```python
from build123d import *

# Parameters (mm, degrees)
F1_DEPTH = 914.4
F2_R     = 19.05
F3_DEPTH = 127
F4_W     = 41.148
F4_H     = 203.2
F5_DEPTH = 127


with BuildPart() as f1:
    # F0 (on Front) → F1 (new body, symmetric)
    with BuildSketch(Plane.XZ):
        with BuildLine():
            ThreePointArc((50.8, 44.45), (48.940128, 48.940128), (44.45, 50.8))
            Line((44.45, 50.8), (-44.45, 50.8))
            ThreePointArc((-44.45, 50.8), (-48.940128, 48.940128), (-50.8, 44.45))
            Line((-50.8, 44.45), (-50.8, -44.45))
            ThreePointArc((-50.8, -44.45), (-48.940128, -48.940128), (-44.45, -50.8))
            Line((-44.45, -50.8), (44.45, -50.8))
            ThreePointArc((44.45, -50.8), (48.940128, -48.940128), (50.8, -44.45))
            Line((50.8, -44.45), (50.8, 44.45))
        make_face()
        with BuildLine():
            Line((-34.925, 41.275), (34.925, 41.275))
            ThreePointArc((34.925, 41.275), (39.415128, 39.415128), (41.275, 34.925))
            Line((41.275, 34.925), (41.275, -34.925))
            ThreePointArc((41.275, -34.925), (39.415128, -39.415128), (34.925, -41.275))
            Line((34.925, -41.275), (-34.925, -41.275))
            ThreePointArc((-34.925, -41.275), (-39.415128, -39.415128), (-41.275, -34.925))
            Line((-41.275, -34.925), (-41.275, 34.925))
            ThreePointArc((-41.275, 34.925), (-39.415128, 39.415128), (-34.925, 41.275))
        make_face(mode=Mode.SUBTRACT)
    extrude(amount=F1_DEPTH, both=True)

    # F2 (on face) → F3 (cut)
    with BuildSketch(Plane.YZ.offset(50.8)):
        with Locations((304.8, 0)):
            Circle(F2_R)
        with Locations((-762, 0)):
            Circle(F2_R)
        with Locations((-609.6, 0)):
            Circle(F2_R)
        with Locations((-457.2, 0)):
            Circle(F2_R)
        with Locations((-304.8, 0)):
            Circle(F2_R)
        with Locations((-152.4, 0)):
            Circle(F2_R)
        Circle(F2_R)
        with Locations((152.4, 0)):
            Circle(F2_R)
        with Locations((457.2, 0)):
            Circle(F2_R)
        with Locations((609.6, 0)):
            Circle(F2_R)
    extrude(amount=-F3_DEPTH, mode=Mode.SUBTRACT)

    # F4 (on face) → F5 (cut)
    with BuildSketch(Plane.XY.offset(50.8)):
        with Locations((0, 914.4)):
            Rectangle(F4_W, F4_H)
    extrude(amount=-F5_DEPTH, mode=Mode.SUBTRACT)


solid = f1.part
```
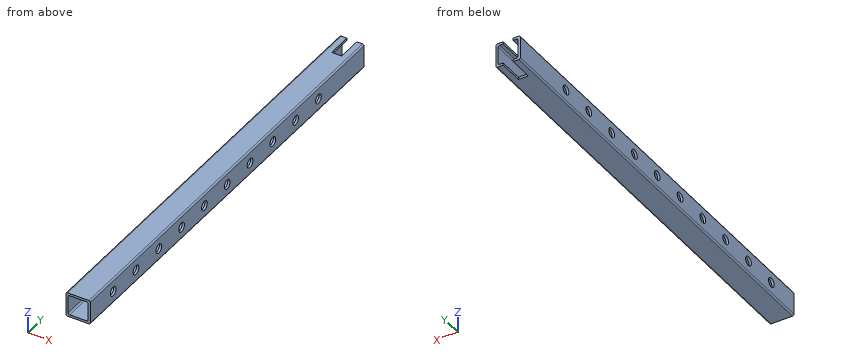
The model under review builds one solid part; all positions refer to its coordinate system, in mm. Round coordinates to 2 decimals unless told otherwise and drop trailing zeros. Order: outer loops, then holes, each group sorted by start corner. A loop starts at its lowest first (then second) coordinate and runs counter-clockwise, first axis right, second up. Notation, with made-up numbers: (57.5, -4.5) - (91.5, -4.5) arc R26 cw to (91.5, 24.5) - close; hole circle Ø5 at (-7, 28.25). An arc over 180 degrees is marked (long way). Answer in a Markdown table with one row per item.
(1) Clearance check with flat-ended pins moving along their axes: P1, Ø23, axis at y = -762, z = 0, coming from the +X side; P2, Ø10.5, axis at x = 2, z = -46.5, coming from the +Y side; P3, Ø3, axis at y = 882.5, z = 47, coming from the -X side. State where each tip first meets the part, or that it passes through.
Result set:
| item | result |
|---|---|
| P1 | passes through |
| P2 | stops at y = 812.8 |
| P3 | stops at x = -50.71 |
(2) For line 1 (X direction, y = -589, z = -31) (3 decimals); line 2 (Z direction, x = 36.5, y = -362), list the stretches that pass through material, from the lowest coordinate up. Write a range as from..to.
Result set:
| item | result |
|---|---|
| line 1 | x = -50.8..-41.275, 41.275..50.8 |
| line 2 | z = -50.8..-41.08, 41.08..50.8 |
(3) Take a section at D-D on z = 0. Count the separate pieces of the cut face and the enclosed holes in it, plus the area to 3 significant figures.
Result set:
| item | result |
|---|---|
| separate pieces | 22 |
| enclosed holes | 0 |
| area | 27,600 mm2 |
(4) Take a section at C-C on y = 191.5. Write out the cut boundary in (x, z) (3 decimals).
Result set:
| item | result |
|---|---|
| outline | (-50.8, -44.45) arc R6.35 ccw to (-44.45, -50.8) - (44.45, -50.8) arc R6.35 ccw to (50.8, -44.45) - (50.8, 44.45) arc R6.35 ccw to (44.45, 50.8) - (-44.45, 50.8) arc R6.35 ccw to (-50.8, 44.45) - close; hole (-41.275, -34.925) arc R6.35 ccw to (-34.925, -41.275) - (34.925, -41.275) arc R6.35 ccw to (41.275, -34.925) - (41.275, 34.925) arc R6.35 ccw to (34.925, 41.275) - (-34.925, 41.275) arc R6.35 ccw to (-41.275, 34.925) - close |
(5) Take a section at A-A on x = -1.5. Write out the cut boundary in (y, z) (3 decimals).
Result set:
| item | result |
|---|---|
| outline | (-914.4, -50.8) - (812.8, -50.8) - (812.8, -41.275) - (-914.4, -41.275) - close; (-914.4, 41.275) - (812.8, 41.275) - (812.8, 50.8) - (-914.4, 50.8) - close |
(6) Take a section at B-B on y = 457.2. Write out the cut boundary in (x, z) (3 decimals), plus the area to 3 significant figures.
Result set:
| item | result |
|---|---|
| outline | (-50.8, -44.45) arc R6.35 ccw to (-44.45, -50.8) - (44.45, -50.8) arc R6.35 ccw to (50.8, -44.45) - (50.8, -19.05) - (41.275, -19.05) - (41.275, -34.925) arc R6.35 cw to (34.925, -41.275) - (-34.925, -41.275) arc R6.35 cw to (-41.275, -34.925) - (-41.275, -19.05) - (-50.8, -19.05) - close; (-50.8, 19.05) - (-41.275, 19.05) - (-41.275, 34.925) arc R6.35 cw to (-34.925, 41.275) - (34.925, 41.275) arc R6.35 cw to (41.275, 34.925) - (41.275, 19.05) - (50.8, 19.05) - (50.8, 44.45) arc R6.35 ccw to (44.45, 50.8) - (-44.45, 50.8) arc R6.35 ccw to (-50.8, 44.45) - close |
| area | 2,780 mm2 |
